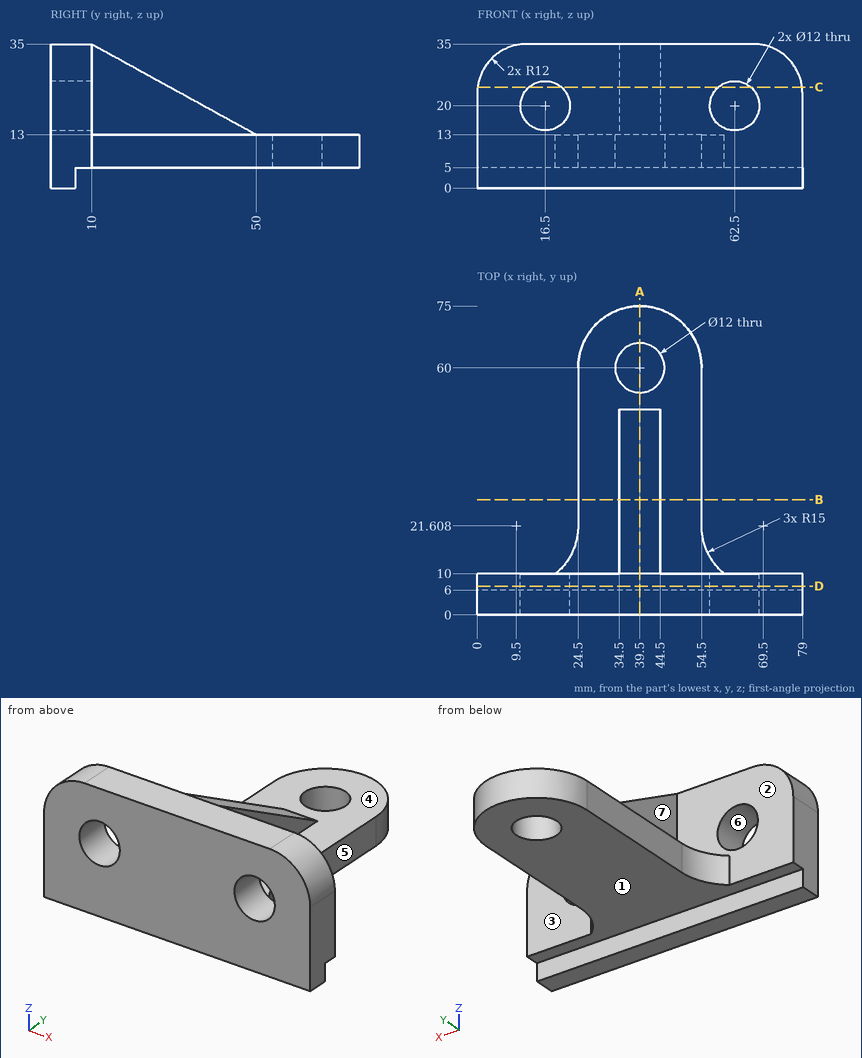
Job drawing, mm, ordinate dimensions from the low corner. One solid piece. A direction names the side the tool comes from. Give positions to 0.01 mm unless a question says otherwise; leave off trailing zeros. Order: outer loops, then holes, each group sorted by start corner. A loop starts at its lowest first (then second) coordinate and runs counter-clockwise, first axis right, second up. Notation, with made-up numbers: (17.5, 6.5) - (71.5, 6.5) arc R27 cw to (71.5, 44.5) - close; hole circle Ø9 at (43, 42). An arc over 180 degrees is marked (long way). Answer in a Markdown table with one row per item.
1. Saw through at D-D, the plane y = 7. Give the cut face in (x, z), plus the area to 3 significant figures.
Data:
| item | result |
|---|---|
| outline | (0, 5) - (79, 5) - (79, 23) arc R12 ccw to (67, 35) - (12, 35) arc R12 ccw to (0, 23) - close; hole circle Ø12 at (16.5, 20); hole circle Ø12 at (62.5, 20) |
| area | 2,080 mm² |
2. Saw through at C-C, the plane z = 24.5. Give the cut face in (x, y).
Data:
| item | result |
|---|---|
| outline | (0.09, 0) - (12.53, 0) - (12.53, 10) - (0.09, 10) - close; (20.47, 0) - (58.53, 0) - (58.53, 10) - (44.5, 10) - (44.5, 29.09) - (34.5, 29.09) - (34.5, 10) - (20.47, 10) - close; (66.47, 0) - (78.91, 0) - (78.91, 10) - (66.47, 10) - close |
3. Flat gauge pins, fed straight in: pin 1 (4 mm diameter, centred on y = 46, z = 11, fed in from -X); pin 2 (17.5 mm diameter, centred on y = 37, z = 21, fed in from +X); pin 3 (5 mm diameter, centred on x = 31, z = 24.5, fed in from +Y); pin 4 (4 mm diameter, centred on x = 47.5, z = 10.5, fed in from -Y). Where does each tip first touch, or does it go through?
Data:
| item | result |
|---|---|
| pin 1 | stops at x = 24.5 |
| pin 2 | stops at x = 54.5 |
| pin 3 | stops at y = 10 |
| pin 4 | stops at y = 0 |
4. Pull direction X, two halves, no side cores. Call the marked faces 5, 6 and 7: pulls with the +X half, pulls with the -X half, needs draft (parallel to the pull), parting line crosses it, or undercut.
Data:
| item | result |
|---|---|
| face 5 | pulls with the +X half |
| face 6 | undercut |
| face 7 | pulls with the -X half |
5. Saw through at A-A, the plane x = 39.5. Give the cut face in (y, z).
Data:
| item | result |
|---|---|
| outline | (0, 0) - (6, 0) - (6, 5) - (54, 5) - (54, 13) - (50, 13) - (10, 35) - (0, 35) - close; (66, 5) - (75, 5) - (75, 13) - (66, 13) - close |
6. Saw through at B-B, the plane y = 28. Give the cut face in (x, z).
Data:
| item | result |
|---|---|
| outline | (24.5, 5) - (54.5, 5) - (54.5, 13) - (44.5, 13) - (44.5, 25.1) - (34.5, 25.1) - (34.5, 13) - (24.5, 13) - close |
7. Probe probe 1 along X at (y, z) = (7, 20); probe 2 along Z at (x, y) = (62, 4); probe 3 along Y at (x, z) = (39.5, 9.25). List the from-to ranges inside material, lowest first. Write a range as [from, to].
Data:
| item | result |
|---|---|
| probe 1 | x = [0, 10.5], [22.5, 56.5], [68.5, 79] |
| probe 2 | z = [0, 14.02], [25.98, 35] |
| probe 3 | y = [0, 54], [66, 75] |
8. Tool access for the marked faces 1, 2, 3 and 4: list every direction of +Z, -Z, +X, -X, +Y, -Y with a clear straight run to the whole face (end or side of a thin tool).
Data:
| item | result |
|---|---|
| face 1 | -Z, +X, -X, +Y |
| face 2 | +Z, -X, +Y |
| face 3 | +Z, +X, +Y |
| face 4 | +Z, +Y |
